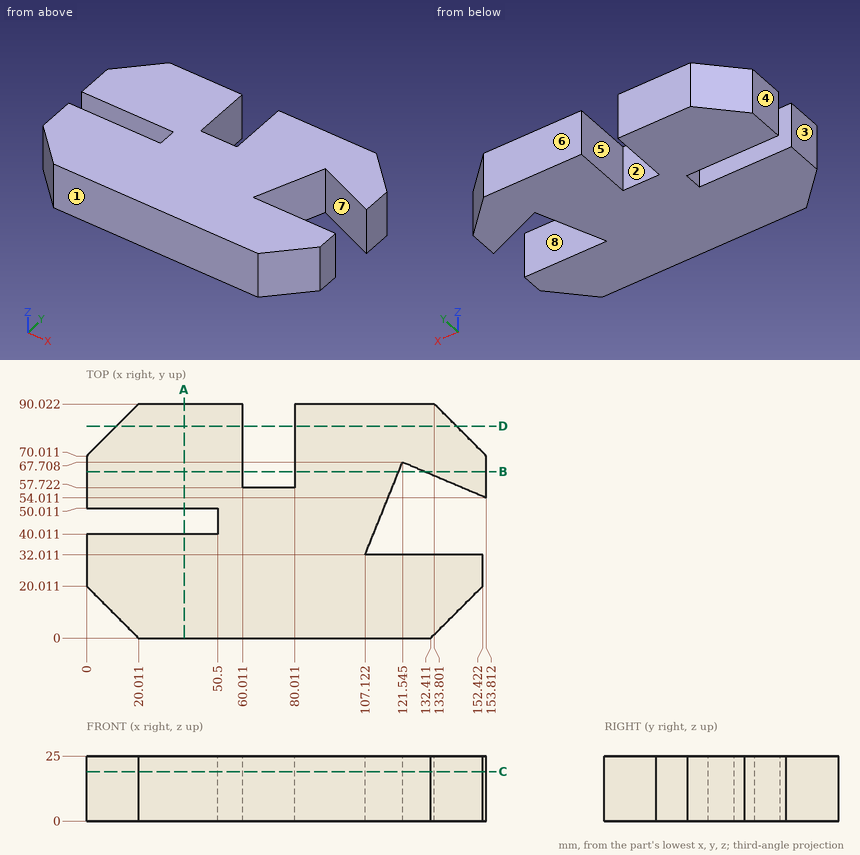
For this review, use the dimensioned drawing (mm, ordinates from the lowest corner) and the shaded views. A direction names the side the tool comes from. Give positions to 0.01 mm unless a question says otherwise; leave off trailing zeros. Order: outer loops, then holes, each group sorted by start corner. A loop starts at its lowest first (then second) coordinate and runs counter-clockwise, first axis right, second up. Notation, with made-up numbers: (6.25, 1.25) -> (60.25, 1.25) arc R20 cw to (60.25, 27.25) -> close; hole circle Ø10 at (11, 74.25). An arc over 180 degrees is marked (long way). Write item = value, one per line. Start each with the question number.
(1) Draft analysis for pull direction X (two halves, no side actions). For the marked faces 1, 2 and 3, state which applies: +X half, -X half, draft (parallel to the pull), parting line (faces both ways), or undercut.
(2) For L1, parallel to Y at x = 23, z = 10.5; L2, parallel to X at y = 62.5, z = 12 (1 decimal); L3, parallel to X at y = 58.5, z = 18.75 (1 decimal), list the stretches that pass through material, from the lowest coordinate up. Write a range as from..to.
(3) Take a section at B-B (y = 64). Write out the cut boundary in (x, z), plus the area to 3 significant figures.
(4) Take a section at D-D (y = 81.5). Write out the cut boundary in (x, z).
(5) Take a section at A-A (x = 37.5). Write out the cut boundary in (y, z), plus the area to 3 significant figures.
(6) Take a section at C-C (z = 19). Write out the cut boundary in (x, y) (1 decimal).
(7) Tool access review of the marked faces 4, 5, 6, 7 and 8: name each direction out of +Z, -Z, +X, -X, +Y, -Y from which nothing blocks a thin tool from reaching the whole face with its end or side.
(8) For pin 1 Ø5 at (y, z) = (11, 20.5) entering from -X; pin 2 Ø13 at (y, z) = (27.5, 9.5) entering from +X; pin 3 Ø8 at (y, z) = (45.5, 11.5) entering from -X, all flat-tipped, find the tip position at first contact; note any pin that passes through.
Returned:
q1.face_1 = draft
q1.face_2 = undercut
q1.face_3 = -X half
q2.L1 = 0..40.01, 50.01..90.02
q2.L2 = 0..60, 80..119.4, 133.8..153.8
q2.L3 = 0..60, 80..117.8, 143.2..153.8
q3.outline = (0, 0) -> (60.01, 0) -> (60.01, 25) -> (0, 25) -> close; (80.01, 0) -> (120.05, 0) -> (120.05, 25) -> (80.01, 25) -> close; (130.28, 0) -> (153.81, 0) -> (153.81, 25) -> (130.28, 25) -> close
q3.area = 3,090 mm²
q4.outline = (11.49, 0) -> (60.01, 0) -> (60.01, 25) -> (11.49, 25) -> close; (80.01, 0) -> (142.32, 0) -> (142.32, 25) -> (80.01, 25) -> close
q5.outline = (0, 0) -> (40.01, 0) -> (40.01, 25) -> (0, 25) -> close; (50.01, 0) -> (90.02, 0) -> (90.02, 25) -> (50.01, 25) -> close
q5.area = 2,000 mm²
q6.outline = (0, 20) -> (20, 0) -> (132.4, 0) -> (152.4, 20) -> (152.4, 32) -> (107.1, 32) -> (121.5, 67.7) -> (153.8, 54) -> (153.8, 70) -> (133.8, 90) -> (80, 90) -> (80, 57.7) -> (60, 57.7) -> (60, 90) -> (20, 90) -> (0, 70) -> (0, 50) -> (50.5, 50) -> (50.5, 40) -> (0, 40) -> close
q7.face_4 = +Z, -Z, -X, +Y, -Y
q7.face_5 = +Z, -Z, +Y
q7.face_6 = +Z, -Z, +X, -X, +Y
q7.face_7 = +Z, -Z
q7.face_8 = +Z, -Z, +X
q8.pin_1 = 6.51
q8.pin_2 = 152.42
q8.pin_3 = 50.5
